Geometry check sheet. Reference: the model listing, model coordinates, mm. Face numbers are marked on the shaded views. Round coordinates to 2 decimals unless told otherwise and drop trailing zeros. Order: outer loops, then holes, each group sorted by start corner. A loop starts at its lowest first (then second) coordinate and runs counter-clockwise, first axis right, second up.
(1) Sectioned sample at C-C (x = 2060). Record the boundary of the cut face in (y, z), plus the area to 3 significant figures.
(2) Release check for a two-part mould opening along Z. For the marked faces 1, 2 and 3 record: +Z half, -Z half, draft (parallel to the pull), parting line (faces both ways), or undercut.
(3) Sectioned sample at B-B (z = 105). Record the boundary of the cut face in (x, y).
(4) Go/stop test with flat-tipped pins: pin 1 (2 mm diameter, centred on y = 6, z = 106.5, fed in from -X); pin 2 (5 mm diameter, centred on x = 2058.5, y = 11.5, fed in from +Z); pin 3 (6 mm diameter, centred on y = 4, z = 84, fed in from +X). Record where each tip stops, or that it passes through.
(5) Sectioned sample at A-A (y = 21.75). Record the boundary of the cut face in (x, z).
(6) Material ranges on line 1 along X through (y, z) = (7, 116.5); line 2 along X through (y, z) = (13, 115); line 3 along Z through (x, y) = (2060.75, 12), recorded low to high.
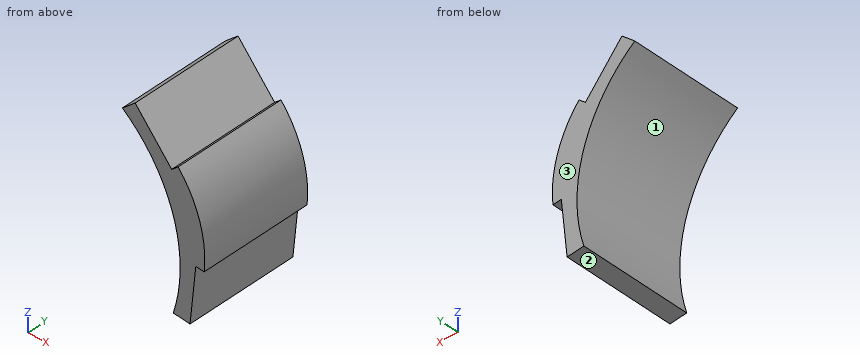
Autodesk Fusion 360 part; units mm, degrees
sketch "Front Most Corner" plane through (0, 0, 0) normal (0, 1, 0) x (1, 0, 0)
  circle A0 centre (2048.0968, -93.3767) radius 25 construction
  line L0 (1842.0683, -371.981) -> (2073.5797, -102.0665)
  line L1 (2073.9927, -100.7451) -> (2060.9213, 25.5804)
  line L2 (2072.964, -90.8036) -> (2048.0968, -93.3767) construction
  line L3 (2072.964, -90.8036) -> (2071.0691, -90.9997)
  line L4 (2071.0691, -90.9997) -> (2069.762, -78.3671)
  line L5 (2069.762, -78.3671) -> (2065.9722, -78.7593)
  line L6 (2067.0728, -109.6528) -> (2065.6268, -108.4126)
  line L7 (2065.6268, -108.4126) -> (2057.3585, -118.0524)
  arc A1 (2067.0728, -109.6528) -> (2072.964, -90.8036) centre (2048.0968, -93.3767) ccw
  line L8 (2057.3585, -118.0524) -> (2054.4666, -115.5719)
  line L9 (2048.0968, -93.3767) -> (2071.9585, -100.8346) construction
  arc A2 (2054.4666, -115.5719) -> (2065.9722, -78.7593) centre (2033.7666, -88.8979) ccw
  point P0 (2065.993, -98.9701)
  dimension "d1" = 50
  dimension "d2" = 25
  dimension "d3" = 25
extrude "Extrude1" add sketch "Front Most Corner" along normal blind 25.4
Answer below:
1. outline: (0, 110.15) - (25.4, 110.15) - (25.4, 114.97) - (0, 114.97) - close
1. area: 122 mm2
2. face 1: undercut
2. face 2: -Z half
2. face 3: draft
3. outline: (2063.44, 0) - (2070.23, 0) - (2070.23, 25.4) - (2063.44, 25.4) - close
4. pin 1: stops at x = 2061.94
4. pin 2: stops at z = 118.05
4. pin 3: stops at x = 2070.66
5. outline: (2054.47, 115.57) arc R33.76 cw to (2065.97, 78.76) - (2069.76, 78.37) - (2071.07, 91) - (2072.96, 90.8) arc R25 ccw to (2067.07, 109.65) - (2065.63, 108.41) - (2057.36, 118.05) - close
6. line 1: x = 2055.55 to 2058.69
6. line 2: x = 2055.18 to 2059.98
6. line 3: z = 109.19 to 114.1
